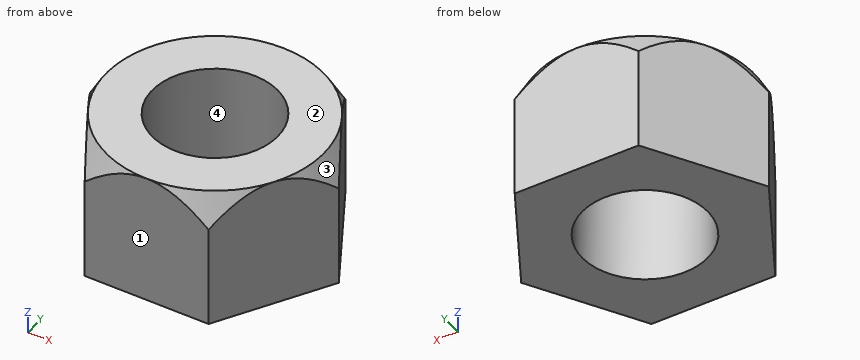
```python
from build123d import *

# Parameters (mm, degrees)
F0_R     = 12
F1_DEPTH = 25


with BuildPart() as f1:
    # F0 (on Top) → F1 (new body)
    with BuildSketch(Plane.XY):
        Polygon((24, 0), (12, 20.78461), (-12, 20.78461), (-24, 0), (-12, -20.78461), (12, -20.78461), align=None)
        Circle(F0_R, mode=Mode.SUBTRACT)
    extrude(amount=F1_DEPTH)

    # F3 (on Front) → F4 (revolve, cut)
    with BuildSketch(Plane.XZ):
        Polygon((24, 25), (20.78461, 25), (24, 19.430781), align=None)
    revolve(axis=Axis((0, 0, 14.01754), (0, 0, 1)), mode=Mode.SUBTRACT)


solid = f1.part
```
Part model, mm, in its own coordinate system. Face numbers are marked on the shaded views. Round coordinates to 2 decimals unless told otherwise and drop trailing zeros. Loops run counter-clockwise (first coordinate to the right, second up) from the corner with the lowest first, then second, coordinate; pieces in that order, holes last.
Item 1: Cut at A-A, the plane z = 4. Give the cut face in (x, y).
Item 2: Drop flat-ended pins along their axis: P1, Ø5, axis at y = 3.5, z = 14, coming from the -X side; P2, Ø1, axis at x = -7.5, y = 14, coming from the -Z side; P3, Ø2, axis at x = 15, z = 13, coming from the +Y side; P4, Ø5, axis at y = 7.5, z = 9.5, coming from the -X side. Give the stop position or say it passes through.
Item 3: Drill centre lines: line 1 (Y direction, x = 0, z = 19); line 2 (X direction, y = 5.5, z = 1.25); line 3 (Y direction, x = -9.5, z = 10.75). Where is each one in solid material? Low to high.
Item 4: Mould opens along Y. For the marked faces 1, 2, 3 and 4 say: +Y half, -Y half, draft (parallel to the pull), parting line (faces both ways), or undercut.
Item 5: Cut at B-B, the plane z = 21.5. Give the cut face in (x, y), then the cut area to 3 significant figures.
A:
1. outline: (-24, 0) - (-12, -20.78) - (12, -20.78) - (24, 0) - (12, 20.78) - (-12, 20.78) - close; hole circle Ø24 at (0, 0)
2. P1: stops at x = -23.42
2. P2: stops at z = 0
2. P3: stops at y = 17.32
2. P4: stops at x = -21.11
3. line 1: y = -20.78 to -12, 12 to 20.78
3. line 2: x = -20.82 to -10.67, 10.67 to 20.82
3. line 3: y = -20.78 to -7.33, 7.33 to 20.78
4. face 1: -Y half
4. face 2: draft
4. face 3: parting line
4. face 4: undercut
5. outline: (-22.69, -2.26) - (-13.31, -18.52) arc R22.81 ccw to (-9.39, -20.78) - (9.39, -20.78) arc R22.81 ccw to (13.31, -18.52) - (22.69, -2.26) arc R22.81 ccw to (22.69, 2.26) - (13.31, 18.52) arc R22.81 ccw to (9.39, 20.78) - (-9.39, 20.78) arc R22.81 ccw to (-13.31, 18.52) - (-22.69, 2.26) arc R22.81 ccw to start; hole circle Ø24 at (0, 0)
5. area: 1,030 mm2
